```python
from build123d import *
from build123d.topology import SkipClean

# Parameters (mm, degrees)
EXTRUSION1_DEPTH = 2
EXTRUSION2_REACH = 46.533
ESQUISSE2_R      = 1
ESQUISSE3_R      = 3
ESQUISSE3_R_2    = 2
EXTRUSION3_DEPTH = 2
EXTRUSION4_START = -1
ESQUISSE4_R      = 2
EXTRUSION4_DEPTH = 1


with BuildPart() as part:
    # Esquisse1 → Extrusion1 (new body)
    with BuildSketch(Plane(origin=(0, 0, 0), x_dir=(1, 0, 0), z_dir=(0, 1, 0))):
        with BuildLine():
            Line((-41.28500686, 2.999999015), (-28.299900327, 2.560234019))
            ThreePointArc((-28.299900327, 2.560234019), (-25.826566394, 0.001717984), (-28.299900327, -2.55679805))
            Line((-28.299900327, -2.55679805), (-41.28500686, -2.996563046))
            ThreePointArc((-41.28500686, -2.996563046), (-44.386549273, 0.001717984), (-41.28500686, 2.999999015))
        make_face()
    extrude(amount=EXTRUSION1_DEPTH)

    # Esquisse2 → Extrusion2 (cut, up to next)
    with BuildSketch(Plane(origin=(0, 2, 0), x_dir=(-1, 0, 0), z_dir=(0, 1, 0)), mode=Mode.PRIVATE) as extrusion2_sk1:
        with Locations(Location((34.386549273, -0.001717984, 0), (0, 0, 90))):
            Circle(ESQUISSE2_R)
    extrusion2_tool1 = extrude(extrusion2_sk1.sketch, amount=-EXTRUSION2_REACH, mode=Mode.PRIVATE) & part.part
    # Esquisse2 → Extrusion2 (cut, up to next)
    with BuildSketch(Plane(origin=(0, 2, 0), x_dir=(-1, 0, 0), z_dir=(0, 1, 0)), mode=Mode.PRIVATE) as extrusion2_sk2:
        with Locations(Location((31.386549273, -0.001717984, 0), (0, 0, 90))):
            Circle(ESQUISSE2_R)
    extrusion2_tool2 = extrude(extrusion2_sk2.sketch, amount=-EXTRUSION2_REACH, mode=Mode.PRIVATE) & part.part
    # Esquisse2 → Extrusion2 (cut, up to next)
    with BuildSketch(Plane(origin=(0, 2, 0), x_dir=(-1, 0, 0), z_dir=(0, 1, 0)), mode=Mode.PRIVATE) as extrusion2_sk3:
        with Locations(Location((28.386549273, -0.001717984, 0), (0, 0, 90))):
            Circle(ESQUISSE2_R)
    extrusion2_tool3 = extrude(extrusion2_sk3.sketch, amount=-EXTRUSION2_REACH, mode=Mode.PRIVATE) & part.part
    add(extrusion2_tool1.solids().sort_by_distance((-34.386549, 2, -0.001718))[0], mode=Mode.SUBTRACT)
    add(extrusion2_tool2.solids().sort_by_distance((-31.386549, 2, -0.001718))[0], mode=Mode.SUBTRACT)
    add(extrusion2_tool3.solids().sort_by_distance((-28.386549, 2, -0.001718))[0], mode=Mode.SUBTRACT)

    # Esquisse3 → Extrusion3 (add)
    with SkipClean():  # the faces are left unmerged after this step: merging them gives an invalid solid
        with BuildSketch(Plane(origin=(0, 2, 0), x_dir=(1, 0, 0), z_dir=(0, 1, 0))):
            with Locations(Location((-41.386549273, 0.001717984, 0), (0, 0, 88.060312285))):
                Circle(ESQUISSE3_R)
            with Locations(Location((-41.386549273, 0.001717984, 0), (0, 0, 270))):
                Circle(ESQUISSE3_R_2, mode=Mode.SUBTRACT)
        extrude(amount=EXTRUSION3_DEPTH)

    # Esquisse4 → Extrusion4 (cut)
    with SkipClean():  # the faces are left unmerged after this step: merging them gives an invalid solid
        with BuildSketch(Plane(origin=(0, 2, 0), x_dir=(1, 0, 0), z_dir=(0, 1, 0)).offset(EXTRUSION4_START)):
            with Locations(Location((-41.386549273, 0.001717984, 0), (0, 0, 270))):
                Circle(ESQUISSE4_R)
        extrude(amount=EXTRUSION4_DEPTH, mode=Mode.SUBTRACT)


solid = part.part
```
Input: part model. Units: mm. Frame: model coordinates. A direction names the side the tool comes from. Coordinates: 2 decimals unless noted, no trailing zeros. Write each loop counter-clockwise with the first axis right and the second up, starting at its lowest first coordinate (ties: lowest second). Pieces come first, ordered by that corner, then holes. Notation, with made-up numbers: M -30,-19.75 L 23,-19.75 A27 ccw 23,2.25 Z; hole C 21,-36.5 d8. An arc over 180 degrees is marked long. Use one line per item in the form item = value.
Q1. Section C-C (x = -29). Return loops of the section in (y, z), plus the area to 3 significant figures.
Answer below:
outline = M 0,-2.58 L 2,-2.58 L 2,-0.79 L 0,-0.79 Z; M 0,0.79 L 2,0.79 L 2,2.58 L 0,2.58 Z
area = 7.17 mm²
Q2. First-contact query: pin 1 (1.8 mm diameter, centred on x = -31.39, z = 0, fed in from -Y); pin 2 (2.5 mm diameter, centred on x = -34.39, z = 0, fed in from +Y); pin 3 (1 mm diameter, centred on x = -30.5, y = 1, fed in from +Z); pin 4 (3 mm diameter, centred on x = -41.5, z = 0, fed in from +Y). Flat tips, straight axial feed; report the tip coordinate or a pass-through.
Answer below:
pin_1 = through
pin_2 = 2
pin_3 = 2.65
pin_4 = 1
Q3. Set-up query: faces 5 (the face through (-43.16, 2.48, 0.92)), 6 (the face through (-39, 4, -1)). Return all of +Z, -Z, +X, -X, +Y, -Y with unobstructed straight access to the full face (end or side cutting, diameter ignored); none if empty.
Answer below:
face_5 = +Y
face_6 = +Z, -Z, +X, -X, +Y
Q4. Material intervals for probe 1 along X at (y, z) = (1.3, -0.5); probe 2 along Y at (x, z) = (-42.25, -0.5); probe 3 along Y at (x, z) = (-39.25, -2.75), sorted ascending. Write a range as from..to.
Answer below:
probe_1 = -44.34..-43.32, -39.45..-35.25, -33.52..-32.25, -30.52..-29.25, -27.52..-25.88
probe_2 = 0..1
probe_3 = 0..2
Q5. Section B-B (y = 1.3). Return loops of the section in (x, z) (3 decimals).
Answer below:
outline = M -41.285,-3 L -28.3,-2.56 A2.56 ccw -28.3,2.557 L -41.285,2.997 A3 ccw long Z; hole C -41.387,-0.002 d4; hole C -34.387,-0.002 d2; hole C -31.387,-0.002 d2; hole C -28.387,-0.002 d2
Q6. Draft query along Z for faces 1 (the face through (-30.395, 1.014, -0.132)), 2 (the face through (-25.827, 0.986, -0.057)), 3 (the face through (-27.395, 1.014, -0.132)), 4 (the face through (-37, 0, 0)). Return one class per face: released by +Z, released by -Z, zero draft, split by the parting line, or undercut.
Answer below:
face_1 = undercut
face_2 = split by the parting line
face_3 = undercut
face_4 = zero draft
Q7. Section A-A (z = -0.5). Return loops of the section in (x, y), plus the area to 3 significant figures.
Answer below:
outline = M -44.34,0 L -35.25,0 L -35.25,2 L -38.43,2 L -38.43,4 L -39.45,4 L -39.45,1 L -43.32,1 L -43.32,4 L -44.34,4 Z; M -33.52,0 L -32.25,0 L -32.25,2 L -33.52,2 Z; M -30.52,0 L -29.25,0 L -29.25,2 L -30.52,2 Z; M -27.52,0 L -25.88,0 L -25.88,2 L -27.52,2 Z
area = 26.7 mm²
Q8. Section D-D (z = 1.25). Return loops of the section in (x, y).
Answer below:
outline = M -44.11,0 L -26.15,0 L -26.15,2 L -38.66,2 L -38.66,4 L -39.83,4 L -39.83,1 L -42.95,1 L -42.95,4 L -44.11,4 Z
